from build123d import *

# Parameters (mm, degrees)
CROQUIS1_W               = 108
CROQUIS1_H               = 71
SALIENTE_EXTRUIR1_DEPTH  = 1.5
CROQUIS2_W               = 12
CROQUIS2_H               = 3
CROQUIS2_W_2             = 8
CORTAR_EXTRUIR1_DEPTH    = 3
CROQUIS6_W               = 3
CROQUIS6_H               = 14
CROQUIS6_H_2             = 8
CORTAR_EXTRUIR3_DEPTH    = 3
CROQUIS8_W               = 8
CROQUIS8_H               = 3
SALIENTE_EXTRUIR2_DEPTH  = 3
REDONDEO2_R              = 3
CROQUIS9_R               = 1.5
CORTAR_EXTRUIR5_DEPTH    = 3
REDONDEO2_OF_SIMETR_A1_R = 3
CROQUIS10_R              = 4.6
CROQUIS10_R_2            = 3.5
CROQUIS10_R_3            = 2
CROQUIS10_W              = 4.5
CROQUIS10_H              = 7
CORTAR_EXTRUIR6_DEPTH    = 10
CROQUIS12_W              = 13.122983438
CROQUIS12_H              = 10
CROQUIS12_W_2            = 12.481361742
CORTAR_EXTRUIR7_DEPTH    = 10


with BuildPart() as part:
    # Croquis1 → Saliente-Extruir1 (new, symmetric)
    with BuildSketch(Plane(origin=(0, 0, 0), x_dir=(0, 0, -1), z_dir=(1, 0, 0))):
        Rectangle(CROQUIS1_W, CROQUIS1_H)
    extrude(amount=SALIENTE_EXTRUIR1_DEPTH, both=True)

    # Croquis2 → Cortar-Extruir1 (cut)
    with BuildSketch(Plane.ZY.offset(1.5)):
        with Locations((-48, -34)):
            Rectangle(CROQUIS2_W, CROQUIS2_H)
        with Locations((-24, -34)):
            Rectangle(CROQUIS2_W_2, CROQUIS2_H)
        with Locations((-8, -34)):
            Rectangle(CROQUIS2_W_2, CROQUIS2_H)
        with Locations((8, -34)):
            Rectangle(CROQUIS2_W_2, CROQUIS2_H)
        with Locations((24, -34)):
            Rectangle(CROQUIS2_W_2, CROQUIS2_H)
        with Locations((48, -34)):
            Rectangle(CROQUIS2_W, CROQUIS2_H)
        with Locations((48, 34)):
            Rectangle(CROQUIS2_W, CROQUIS2_H)
        with Locations((24, 34)):
            Rectangle(CROQUIS2_W_2, CROQUIS2_H)
        with Locations((8, 34)):
            Rectangle(CROQUIS2_W_2, CROQUIS2_H)
        with Locations((-8, 34)):
            Rectangle(CROQUIS2_W_2, CROQUIS2_H)
        with Locations((-24, 34)):
            Rectangle(CROQUIS2_W_2, CROQUIS2_H)
        with Locations((-48, 34)):
            Rectangle(CROQUIS2_W, CROQUIS2_H)
    extrude(amount=-CORTAR_EXTRUIR1_DEPTH, mode=Mode.SUBTRACT)

    # Croquis6 → Cortar-Extruir3 (cut)
    with BuildSketch(Plane.ZY.offset(1.5)):
        with Locations((52.5, -28.5)):
            Rectangle(CROQUIS6_W, CROQUIS6_H)
        with Locations((52.5, -6.5)):
            Rectangle(CROQUIS6_W, CROQUIS6_H_2)
        with Locations((52.5, 6.5)):
            Rectangle(CROQUIS6_W, CROQUIS6_H_2)
        with Locations((52.5, 28.5)):
            Rectangle(CROQUIS6_W, CROQUIS6_H)
    extrude(amount=-CORTAR_EXTRUIR3_DEPTH, mode=Mode.SUBTRACT)

    # Croquis8 → Saliente-Extruir2 (add)
    with BuildSketch(Plane.ZY.offset(1.5)):
        with Locations((16, 37)):
            Rectangle(CROQUIS8_W, CROQUIS8_H)
    saliente_extruir2 = extrude(amount=-SALIENTE_EXTRUIR2_DEPTH)

    # Redondeo2
    redondeo2_edges = [part.edges().sort_by_distance(p)[0] for p in [
        (0, 38.5, 12),
        (0, 38.5, 20),
    ]]
    fillet(redondeo2_edges, radius=REDONDEO2_R)

    # Croquis9 → Cortar-Extruir5 (cut)
    with BuildSketch(Plane.ZY.offset(1.5)):
        with Locations((16, 34)):
            Circle(CROQUIS9_R)
    cortar_extruir5 = extrude(amount=-CORTAR_EXTRUIR5_DEPTH, mode=Mode.SUBTRACT)

    # Simetría1: Saliente-Extruir2, Cortar-Extruir5 across plane
    add(saliente_extruir2.mirror(Plane.ZX))
    add(cortar_extruir5.mirror(Plane.ZX), mode=Mode.SUBTRACT)

    # Redondeo2 of Simetría1
    redondeo2_of_simetr_a1_edges = [part.edges().sort_by_distance(p)[0] for p in [
        (0, -38.5, 12),
        (0, -38.5, 20),
    ]]
    fillet(redondeo2_of_simetr_a1_edges, radius=REDONDEO2_OF_SIMETR_A1_R)

    # Croquis10 → Cortar-Extruir6 (cut)
    with BuildSketch(Plane.ZY.offset(1.5)):
        with Locations((-25.2, -13.25)):
            Circle(CROQUIS10_R)
        with Locations((-14.4, -13.25)):
            Circle(CROQUIS10_R_2)
        with Locations((-4.6, -22)):
            Circle(CROQUIS10_R_3)
        with Locations((-4.6, -4.5)):
            Circle(CROQUIS10_R_3)
        with Locations((6.85, -13.25)):
            Rectangle(CROQUIS10_W, CROQUIS10_H)
    extrude(amount=-CORTAR_EXTRUIR6_DEPTH, mode=Mode.SUBTRACT)

    # Croquis12 → Cortar-Extruir7 (cut)
    with BuildSketch(Plane.ZY.offset(1.5)):
        with Locations((-31.1, -27.5)):
            Rectangle(CROQUIS12_W, CROQUIS12_H)
        with Locations((36.9, -27.5)):
            Rectangle(CROQUIS12_W_2, CROQUIS12_H)
    extrude(amount=-CORTAR_EXTRUIR7_DEPTH, mode=Mode.SUBTRACT)


solid = part.part
The listing builds one solid part. Answer for the finished solid, in the listing's coordinates (mm). A direction names the side the tool comes from. Coordinates: 2 decimals unless noted, no trailing zeros. Write each loop counter-clockwise with the first axis right and the second up, starting at its lowest first coordinate (ties: lowest second). Pieces come first, ordered by that corner, then holes. Notation, with made-up numbers: M 89.5,5 L 145.5,5 A29 cw 145.5,31 Z; hole C 57,33.25 d5. An arc over 180 degrees is marked long. Write each question's results on one line, items separated by ' | '.
Item 1: The part is cut by section A-A on y = -13.25. Determine the outline of the cut face in (x, z).
Answer below:
outline: M -1.5,-54 L 1.5,-54 L 1.5,-29.8 L -1.5,-29.8 Z; M -1.5,-20.6 L 1.5,-20.6 L 1.5,-17.9 L -1.5,-17.9 Z; M -1.5,-10.9 L 1.5,-10.9 L 1.5,4.6 L -1.5,4.6 Z; M -1.5,9.1 L 1.5,9.1 L 1.5,54 L -1.5,54 Z
Item 2: Given P1, Ø1, axis at x = -1, z = 5, coming from the +Y side; P2, Ø0.9, axis at x = 0, y = -8, coming from the +Z side; P3, Ø0.9, axis at x = 0.5, z = 47.5, coming from the -Y side; P4, Ø2.5, axis at y = 34, z = 16, coming from the -X side, each flat-ended and moving along its own axis, determine where each tip first touches the part or whether it passes through.
Answer below:
P1: y = 32.5 | P2: z = 51 | P3: y = -32.5 | P4: through
Item 3: For a pull along Z with two mould halves and no side action, classify faces 6 (the face through (0, -32.5, 47)), 7 (the face through (0, -34, 42)), 8 (the face through (0, -16.75, 7)) as released by +Z, released by -Z, zero draft, split by the parting line, or undercut.
Answer below:
face 6: zero draft | face 7: released by +Z | face 8: undercut
Item 4: Consider probe 1 along Y at (x, z) = (0.65, 16); probe 2 along Y at (x, z) = (0.3, -4.6); probe 3 along Z at (x, y) = (-0.9, -34). Determine where each line is inside the solid, lowest interval first. Write a range as [from, to].
Answer below:
probe 1: [-38.5, -35.5], [-32.5, 32.5], [35.5, 38.5] | probe 2: [-32.5, -24], [-20, -6.5], [-2.5, 32.5] | probe 3: [-42, -28], [-20, -12], [-4, 4], [12, 14.5], [17.5, 20], [28, 42]
Item 5: Which of the six approach directions +Z, -Z, +X, -X, +Y, -Y give full straight-line access (tool end or side, diameter ignored) to faces 1 (the face through (0, 34, -28)), 2 (the face through (0, 35.5, 0)), 3 (the face through (0, -13, 4.6)), 4 (the face through (0, -35.5, 0)), 5 (the face through (0, -34, 20))?
Answer below:
face 1: +X, -X, +Y | face 2: -Z, +X, -X, +Y | face 3: +X, -X | face 4: -Z, +X, -X, -Y | face 5: +X, -X, -Y
Item 6: The part is cut by section D-D on x = 1.05. State how many separate pieces and enclosed holes the cut face has, and give its area (3 significant figures).
Answer below:
separate pieces: 1 | enclosed holes: 7 | area: 6,830 mm2
Item 7: The part is cut by section C-C on y = -4.5. Determine the outline of the cut face in (x, z).
Answer below:
outline: M -1.5,-54 L 1.5,-54 L 1.5,-6.6 L -1.5,-6.6 Z; M -1.5,-2.6 L 1.5,-2.6 L 1.5,51 L -1.5,51 Z
Item 8: The part is cut by section B-B on z = -16.5. Determine the outline of the cut face in (x, y), and give its area (3 significant figures).
Answer below:
outline: M -1.5,-35.5 L 1.5,-35.5 L 1.5,-16.05 L -1.5,-16.05 Z; M -1.5,-10.45 L 1.5,-10.45 L 1.5,35.5 L -1.5,35.5 Z | area: 196 mm2
